The listing builds one solid part. Answer for the finished solid, in the listing's coordinates (mm). Face numbers are marked on the shaded views. A direction names the side the tool comes from. Give positions to 0.01 mm unless a question says otherwise; leave off trailing zeros. Order: outer loops, then holes, each group sorted by start corner. A loop starts at its lowest first (then second) coordinate and runs counter-clockwise, first axis right, second up. Notation, with made-up numbers: (56, -34.5) - (89, -34.5) arc R22 cw to (89, -23.5) - close; hole circle Ø4 at (2.5, 23.5). An arc over 180 degrees is marked (long way). Answer as a JSON object with one key per item and string values. Group by question number.
Q1. A cutting plane is placed at A-A, the plane y = 0. Give the vertices of the cut face in (x, z).
Q2. A cutting plane is placed at C-C, the plane z = 30.5. Give the vertices of the cut face in (x, y) (1 decimal).
Q3. Given pin 1 (3 mm diameter, centred on y = -2.5, z = 16.5, fed in from +X); pin 2 (2 mm diameter, centred on x = 7.5, z = 6, fed in from -Y); pin 3 (5.5 mm diameter, centred on x = -11.29, y = -31.01, fed in from +Z); pin 4 (3 mm diameter, centred on x = 32.5, y = 5.73, fed in from -Z), each flat-ended and moving along its own axis, determine where each tip first touches the part or whether it passes through.
Q4. A cutting plane is placed at B-B, the plane x = 0. Give the vertices of the cut face in (y, z).
Q5. A cutting plane is placed at D-D, the plane y = 33. Give the vertices of the cut face in (x, z).
Q6. The mould has two halves that part along Y. Classify the marked faces 3, 4 and 5: released by +Y, released by -Y, zero draft, split by the parting line, or undercut.
Q7. For the marked faces 1 and 2, determine the directions among +Z, -Z, +X, -X, +Y, -Y from which every point of the face is accessible in a straight line to the end or side of a thin tool.
Q8. Consider line 1 (X direction, y = -28.5, z = 8.5); line 2 (X direction, y = -16.5, z = 4.5); line 3 (Y direction, x = -21, z = 3). Determine where each line is inside the solid, lowest interval first.
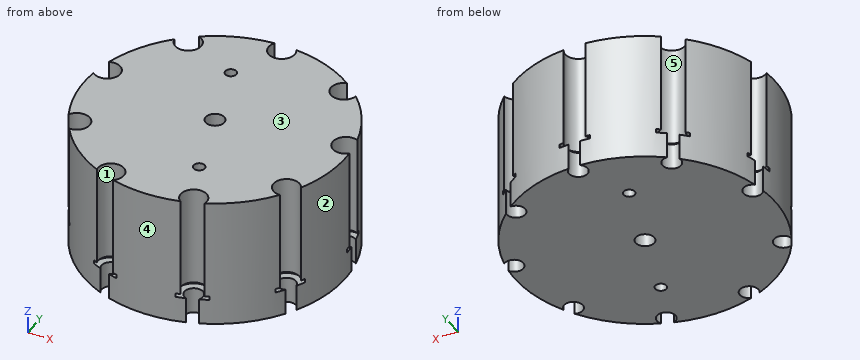
from build123d import *

# Parameters (mm, degrees)
SKETCH_1_R               = 35
SKETCH_1_R_2             = 2.5
EXTRUDE_1_DEPTH          = 35
SKETCH_2_R               = 3.5
CUT_EXTRUDE_1_DEPTH      = 27
SKETCH_3_R               = 2.5
CUT_EXTRUDE_2_DEPTH      = 8
SKETCH_5_R               = 4.5
CUT_EXTRUDE_3_DEPTH      = 1
PATTERN_CIRCULAR_1_COUNT = 9
SKETCH_6_R               = 1.5
CUT_EXTRUDE_4_DEPTH      = 35


with BuildPart() as part:
    # 草图1 → 凸台-拉伸1 (new body)
    with BuildSketch(Plane.XY):
        Circle(SKETCH_1_R)
        Circle(SKETCH_1_R_2, mode=Mode.SUBTRACT)
    extrude(amount=EXTRUDE_1_DEPTH)

    # 草图2 → 切除-拉伸1 (cut)
    with BuildSketch(Plane.XY.offset(35)):
        with Locations((0, 33)):
            Circle(SKETCH_2_R)
    cut_extrude_1 = extrude(amount=-CUT_EXTRUDE_1_DEPTH, mode=Mode.SUBTRACT)

    # 草图3 → 切除-拉伸2 (cut)
    with BuildSketch(Plane.XY.offset(8)):
        with Locations((0, 33)):
            Circle(SKETCH_3_R)
    cut_extrude_2 = extrude(amount=-CUT_EXTRUDE_2_DEPTH, mode=Mode.SUBTRACT)

    # 草图5 → 切除-拉伸3 (cut)
    with BuildSketch(Plane.XY.offset(8)):
        with Locations((0, 33)):
            Circle(SKETCH_5_R)
    cut_extrude_3 = extrude(amount=-CUT_EXTRUDE_3_DEPTH, mode=Mode.SUBTRACT)

    # 阵列(圆周)1: 切除-拉伸1, 切除-拉伸2, 切除-拉伸3 ×9 about axis
    pattern_circular_1_axis = Axis((0, 0, 0), (0, 0, 1))
    add([cut_extrude_1.rotate(pattern_circular_1_axis, i * 360 / PATTERN_CIRCULAR_1_COUNT) for i in range(1, PATTERN_CIRCULAR_1_COUNT)], mode=Mode.SUBTRACT)
    add([cut_extrude_2.rotate(pattern_circular_1_axis, i * 360 / PATTERN_CIRCULAR_1_COUNT) for i in range(1, PATTERN_CIRCULAR_1_COUNT)], mode=Mode.SUBTRACT)
    add([cut_extrude_3.rotate(pattern_circular_1_axis, i * 360 / PATTERN_CIRCULAR_1_COUNT) for i in range(1, PATTERN_CIRCULAR_1_COUNT)], mode=Mode.SUBTRACT)

    # 草图6 → 切除-拉伸4 (cut)
    with BuildSketch(Plane(origin=(0, 0, 0), x_dir=(-1, 0, 0), z_dir=(0, 0, -1))):
        with Locations((6.180339887, 19.021130326)):
            Circle(SKETCH_6_R)
        with Locations((-6.180339887, -19.021130326)):
            Circle(SKETCH_6_R)
    extrude(amount=-CUT_EXTRUDE_4_DEPTH, mode=Mode.SUBTRACT)


solid = part.part
Reply:
{
 "1": {"outline": "(-35, 0) - (-2.5, 0) - (-2.5, 35) - (-35, 35) - close; (2.5, 0) - (35, 0) - (35, 35) - (2.5, 35) - close"},
 "2": {"outline": "(-34.9, 3.1) arc R35 ccw to (-31.7, -14.9) arc R3.5 cw (long way) to (-28.7, -20) arc R35 ccw to (-14.7, -31.8) arc R3.5 cw (long way) to (-9.2, -33.8) arc R35 ccw to (9.2, -33.8) arc R3.5 cw (long way) to (14.7, -31.8) arc R35 ccw to (28.7, -20) arc R3.5 cw (long way) to (31.7, -14.9) arc R35 ccw to (34.9, 3.1) arc R3.5 cw (long way) to (33.8, 9) arc R35 ccw to (24.7, 24.8) arc R3.5 cw (long way) to (20.2, 28.6) arc R35 ccw to (3, 34.9) arc R3.5 cw (long way) to (-3, 34.9) arc R35 ccw to (-20.2, 28.6) arc R3.5 cw (long way) to (-24.7, 24.8) arc R35 ccw to (-33.8, 9) arc R3.5 cw (long way) to start; hole circle Ø3 at (-6.2, 19); hole circle Ø5 at (0, 0); hole circle Ø3 at (6.2, -19)"},
 "3": {"pin 1": "stops at x = 34.99", "pin 2": "stops at y = -34.39", "pin 3": "stops at z = 7", "pin 4": "passes through"},
 "4": {"outline": "(-35, 0) - (-2.5, 0) - (-2.5, 35) - (-35, 35) - close; (2.5, 0) - (30.5, 0) - (30.5, 7) - (28.5, 7) - (28.5, 8) - (29.5, 8) - (29.5, 35) - (2.5, 35) - close"},
 "5": {"outline": "(-11.66, 0) - (-2.5, 0) - (-2.5, 7) - (-4.5, 7) - (-4.5, 8) - (-3.5, 8) - (-3.5, 35) - (-11.66, 35) - close; (2.5, 0) - (11.66, 0) - (11.66, 35) - (3.5, 35) - (3.5, 8) - (4.5, 8) - (4.5, 7) - (2.5, 7) - close"},
 "6": {"face 3": "zero draft", "face 4": "released by -Y", "face 5": "undercut"},
 "7": {"face 1": "+Z", "face 2": "+Z, -Z, +X"},
 "8": {"line 1": "x = -20.32 to -13.73, -8.85 to 8.85, 13.73 to 20.32", "line 2": "x = -26.08 to 26.08", "line 3": "y = -28 to 22.79, 27.77 to 28"}
}
